from build123d import *

# Parameters (mm, degrees)
SKETCH1_R               = 6.25
BOSS_EXTRUDE1_DEPTH     = 4
THREAD1_PITCH           = 1
BOSS_EXTRUDE2_DEPTH     = 5
CUT_EXTRUDE1_DEPTH      = 3
CUT_EXTRUDE2_DEPTH      = 13.59546881
CUT_EXTRUDE2_DEPTH_BACK = 13.59546881
SKETCH6_W               = 1.7
SKETCH6_H               = 1.7


with BuildPart() as part:
    # Sketch1 → Boss-Extrude1 (new body)
    with BuildSketch(Plane(origin=(0, 0, 0), x_dir=(1, 0, 0), z_dir=(0, 1, 0))):
        with Locations(Location((0, 0, 0), (0, 0, 270))):
            Circle(SKETCH1_R)
    extrude(amount=BOSS_EXTRUDE1_DEPTH)

    # Thread1: the profile of Thread Profile1 profile screwed along a right-hand helix of 4 turns, 8 arcs to a turn; built about Z, then put on its axis
    thread1_z = Axis((0, 0, 0), (0, 0, 1))
    thread1_corners = [(6.2503, 0, -0.000173205), (6.2503, 0, 0.875173202), (5.708734125, 0, 0.562499999), (5.708734125, 0, 0.312499999)]
    with BuildLine(mode=Mode.PRIVATE) as thread1_profile:
        Line(thread1_corners[0], thread1_corners[1])
        Line(thread1_corners[1], thread1_corners[2])
        Line(thread1_corners[2], thread1_corners[3])
        Line(thread1_corners[3], thread1_corners[0])
    thread1_cap = Face(thread1_profile.wire())
    thread1_turn_angles = [0, 22.5, 45, 67.5, 90, 112.5, 135, 157.5, 180, 202.5, 225, 247.5, 270, 292.5, 315, 337.5, 360]
    thread1_turn_weights = [1, 0.9238795325112867, 1, 0.9238795325112867, 1, 0.9238795325112867, 1, 0.9238795325112867, 1, 0.9238795325112867, 1, 0.9238795325112867, 1, 0.9238795325112867, 1, 0.9238795325112867, 1]
    thread1_turn_rails = [Edge.make_bspline([Vector(p[0], p[1], 0).rotate(thread1_z, thread1_turn_angles[k]) / thread1_turn_weights[k] + Vector(0, 0, p[2] + THREAD1_PITCH * thread1_turn_angles[k] / 360) for k in range(17)], [0, 0, 0, 1, 1, 2, 2, 3, 3, 4, 4, 5, 5, 6, 6, 7, 7, 8, 8, 8], 2, thread1_turn_weights) for p in thread1_corners]
    thread1_turn_sides = [Face.make_surface_from_curves(thread1_turn_rails[p[0]], thread1_turn_rails[p[1]]) for p in [(0, 1), (1, 2), (2, 3), (3, 0)]]
    thread1 = Plane(origin=(0, 4, 0), x_dir=(-1, 0, 0), z_dir=(0, -1, 0)) * Solid(Shell([*[p.moved(Location((0, 0, THREAD1_PITCH * i))) for i in range(4) for p in thread1_turn_sides], thread1_cap, thread1_cap.rotate(thread1_z, 1440).moved(Location((0, 0, THREAD1_PITCH * 1440 / 360)))]))
    add(thread1, mode=Mode.SUBTRACT)

    # Sketch4 → Boss-Extrude2 (add)
    with BuildSketch(Plane(origin=(0, 4, 0), x_dir=(1, 0, 0), z_dir=(0, 1, 0))):
        Polygon((8.371578903, 0), (4.185789452, 7.25), (-4.185789452, 7.25), (-8.371578903, 0), (-4.185789452, -7.25), (4.185789452, -7.25), align=None)
    extrude(amount=BOSS_EXTRUDE2_DEPTH)

    # Sketch5 → Cut-Extrude1 (cut)
    with BuildSketch(Plane(origin=(0, 9, 0), x_dir=(1, 0, 0), z_dir=(0, 1, 0))):
        Polygon((3.031088913, 5.25), (-3.031088913, 5.25), (-6.062177826, 0), (-3.031088913, -5.25), (3.031088913, -5.25), (6.062177826, 0), align=None)
    extrude(amount=-CUT_EXTRUDE1_DEPTH, mode=Mode.SUBTRACT)

    # Sketch6 → Cut-Extrude2 (cut, two sides: drawn at the far end of the back side and taken through both)
    with BuildSketch(Plane(origin=(0, 6, 0), x_dir=(1, 0, 0), z_dir=(0, 1, 0)).offset(-CUT_EXTRUDE2_DEPTH_BACK)):
        Rectangle(SKETCH6_W, SKETCH6_H)
    extrude(amount=CUT_EXTRUDE2_DEPTH + CUT_EXTRUDE2_DEPTH_BACK, mode=Mode.SUBTRACT)


solid = part.part
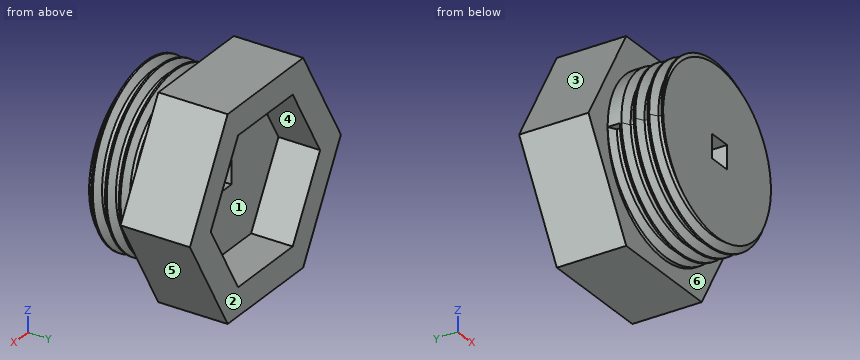
Input: part model. Units: mm. Frame: model coordinates. Face numbers are marked on the shaded views. A direction names the side the tool comes from. Give positions to 0.01 mm unless a question says otherwise; leave off trailing zeros. Write each loop counter-clockwise with the first axis right and the second up, starting at its lowest first coordinate (ties: lowest second). Pieces come first, ordered by that corner, then holes. Notation, with made-up numbers: M 42,13 L 48,13 A22 ccw 48,51 Z; hole C 4.5,39 d1. An arc over 180 degrees is marked long. Use one line per item in the form item = value.
1. First-contact query: P1, Ø3, axis at x = 6.5, y = 2, coming from the -Z side; P2, Ø1, axis at y = 3, z = 4.5, coming from the +X side; P3, Ø0.5, axis at y = 3.5, z = 0, coming from the +X side. Flat tips, straight axial feed; report the tip coordinate or a pass-through.
Outcome:
P1 = -3.72
P2 = 4.65
P3 = 6.25
2. Ray query, L1, parallel to Z at x = 1, y = 7; L2, parallel to Z at x = 0.5, y = 4.25; L3, parallel to Y at x = -2, z = -2.25. Return the intervals inside material, ascending.
Outcome:
L1 = -7.25 to -5.25, 5.25 to 7.25
L2 = -7.25 to -0.85, 0.85 to 7.25
L3 = 0 to 6
3. Cut plane B-B on y = 7.5. Return loops of the section in (x, z).
Outcome:
outline = M -8.37,0 L -4.19,-7.25 L 4.19,-7.25 L 8.37,0 L 4.19,7.25 L -4.19,7.25 Z; hole M -6.06,0 L -3.03,-5.25 L 3.03,-5.25 L 6.06,0 L 3.03,5.25 L -3.03,5.25 Z
4. Cut plane C-C on x = -7.25. Return loops of the section in (y, z), and give its area (3 significant figures).
Outcome:
outline = M 4,-1.94 L 9,-1.94 L 9,1.94 L 4,1.94 Z
area = 19.4 mm²
5. Mould query, pull axis X, two halves, no side actions, for the marked faces 1, 2 and 3. Classes: released by +X, released by -X, zero draft, split by the parting line, or undercut.
Outcome:
face_1 = undercut
face_2 = zero draft
face_3 = released by -X
6. Reachability of the marked faces 4, 5 and 6 from +Z, -Z, +X, -X, +Y, -Y: full face, straight path, thin tool, end or side. Return the list, or none.
Outcome:
face_4 = +Y
face_5 = -Z, +X, +Y, -Y
face_6 = -Y
7. Cut plane A-A on y = 4.75. Return loops of the section in (x, z).
Outcome:
outline = M -8.37,0 L -4.19,-7.25 L 4.19,-7.25 L 8.37,0 L 4.19,7.25 L -4.19,7.25 Z; hole M -0.85,-0.85 L 0.85,-0.85 L 0.85,0.85 L -0.85,0.85 Z
